Autodesk Inventor part; units mm, degrees
ref_plane "scharnier_XY" through (0, -8.75, 0) normal (0, 0, 1) x (1, 0, 0)
ref_plane "scharnier_YZ" through (0, -8.75, 0) normal (1, 0, 0) x (0, 1, 0)
ref_plane "scharnier_ZX" through (0, -8.75, 0) normal (0, 1, 0) x (0, 0, 1)
sketch "Skizze_1" plane through (0, 0, 0) normal (0, 1, 0) x (-1, 0, 0)
  arc A0 (9, 5.9981) -> (8.3959, 7.8036) centre (6, 5.9981) ccw
  line L0 (8.3959, 7.8036) -> (4.8967, 12.4471)
  arc A1 (4.8967, 12.4471) -> (3.9166, 13.2866) centre (2.5008, 10.6417) ccw
  line L1 (3.9166, 13.2866) -> (-0.1415, 15.4588)
  arc A2 (-0.1415, 15.4588) -> (2.0342, 12.1617) centre (-2.1, 11.8) ccw
  line L2 (2.0342, 12.1617) -> (0.5399, 12.031)
  arc A3 (-0.8494, 14.1363) -> (0.5399, 12.031) centre (-2.1, 11.8) ccw
  line L3 (-0.8494, 14.1363) -> (3.5, 11.8082)
  line L4 (3.5, 11.8082) -> (7.5, 6.5)
  line L5 (7.5, 6.5) -> (7.5, 3)
  arc A4 (6, 1.5) -> (7.5, 3) centre (6, 3) ccw
  line L6 (6, 1.5) -> (-5.3, 1.5)
  line L7 (-5.3, 1.5) -> (-6, 0.8)
  line L8 (-6, 0.8) -> (-6, 0)
  line L9 (-6, 0) -> (6, 0)
  arc A5 (6, 0) -> (9, 3) centre (6, 3) ccw
  line L10 (9, 3) -> (9, 5.9981)
extrude "Extrusion1" add sketch "Skizze_1" along normal mid plane 60
sketch "Skizze_2" plane through (0, 0, 0) normal (1, 0, 0) x (0, 1, 0)
  line L0 (8.75, 0) -> (8.75, 1.5)
  line L1 (8.75, 1.5) -> (12.35, 1.5)
  line L2 (12.35, 1.5) -> (10.85, 0)
  line L3 (10.85, 0) -> (8.75, 0)
  line L4 (8.75, 0) -> (8.75, 1.5)
revolve "Revolution1" cut sketch "Skizze_2" angle 360 about axis through (0, 8.75, 0) along (0, 0, -1)
sketch "Skizze_3" plane through (0, 0, 0) normal (1, 0, 0) x (0, 1, 0)
  line L0 (-8.75, 0) -> (-8.75, 1.5)
  line L1 (-8.75, 1.5) -> (-5.15, 1.5)
  line L2 (-5.15, 1.5) -> (-6.65, 0)
  line L3 (-6.65, 0) -> (-8.75, 0)
  line L4 (-8.75, 0) -> (-8.75, 1.5)
revolve "Revolution2" cut sketch "Skizze_3" angle 360 about axis through (0, -8.75, 0) along (0, 0, -1)
sketch "Skizze_5" plane through (0, 0, 0) normal (0, 1, 0) x (-1, 0, 0)
  line L0 (19.1684, 40) -> (-42.1, 40)
  line L1 (-42.1, 40) -> (-42.1, 3)
  line L2 (-42.1, 3) -> (-0.5049, 3)
  line L3 (-0.5049, 3) -> (19.1684, 40)
extrude "Extrusion2" cut sketch "Skizze_5" along normal mid plane 26
ref_plane "scharnier_XY" through (0, -8.75, 0) normal (0, 0, 1) x (1, 0, 0)
ref_plane "scharnier_YZ" through (0, -8.75, 0) normal (1, 0, 0) x (0, 1, 0)
ref_plane "scharnier_ZX" through (0, -8.75, 0) normal (0, 1, 0) x (0, 0, 1)
ref_plane "scharnier_2_XY" through (0, 8.75, 0) normal (0, 0, 1) x (1, 0, 0)
ref_plane "scharnier_2_YZ" through (0, 8.75, 0) normal (1, 0, 0) x (0, 1, 0)
ref_plane "scharnier_2_ZX" through (0, 8.75, 0) normal (0, 1, 0) x (0, 0, 1)
ref_plane "tuer_XY" through (2.1, 0, 11.8) normal (0, 1, 0) x (1, 0, 0)
ref_plane "tuer_YZ" through (2.1, 0, 11.8) normal (1, 0, 0) x (0, 0, -1)
ref_plane "tuer_ZX" through (2.1, 0, 11.8) normal (0, 0, -1) x (0, 1, 0)
properties part number "1XXX_01_04"
The model under review builds one solid part; all positions refer to its coordinate system, in mm. A direction names the side the tool comes from. Give positions to 0.01 mm unless a question says otherwise; leave off trailing zeros. Write each loop counter-clockwise with the first axis right and the second up, starting at its lowest first coordinate (ties: lowest second). Pieces come first, ordered by that corner, then holes.
1. Add section B-B, the plane z = 9.75. Write out the cut boundary in (x, y).
2. Add section A-A, the plane y = -8.75. Write out the cut boundary in (x, z).
3. Add section C-C, the plane y = 14. Write out the cut boundary in (x, z), plus the area to 3 significant figures.
4. Tool access review of faces 4 (the flat face through (-6.671, -0.42, 10.093)), 5 (the flat face through (-1.29, -21.62, 12.99)), 6 (the flat face through (0, 0, 0)), 7 (the flat face through (0, 0, 1.5)), 8 (the flat face through (-4.275, -0.182, 11.99)): name each direction out of +Z, -Z, +X, -X, +Y, -Y from which nothing blocks a thin tool from reaching the whole face with its end or side.
5. Wall thickness on L1, parallel to Y at x = 5.25, z = 9.75; L2, parallel to X at y = -18, z = 10.75; L3, parallel to Z at x = 4.5, y = -24.5: over which ranges is each line inside the solid? List them lowest first.
6. Draft analysis for pull direction Y (two halves, no side actions). For faces 1 (the flat face through (-0.8, -30, 9.2)), 2 (the flat face through (0, -13, 14)), 3 (the cylindrical face through (5.48, 21.38, 9.39)), state which applies: +Y half, -Y half, draft (parallel to the pull), parting line (faces both ways), or undercut.
7. For P1, Ø1, axis at y = 6.5, z = 5, coming from the +X side; P2, Ø0.6, axis at y = -3, z = 0.5, coming from the +X side; P3, Ø3.5, axis at x = -0.5, y = 3, coming from the +Z side, all flat-tipped, find the tip position at first contact; note any pin that passes through.
Worked answers:
1. outline: (-6.93, -30) - (-5.05, -30) - (-5.05, 30) - (-6.93, 30) - close; (-1.51, -30) - (0.42, -30) - (0.42, -13) - (-1.51, -13) - close; (-1.51, 13) - (0.42, 13) - (0.42, 30) - (-1.51, 30) - close; (3.78, -30) - (5.71, -30) - (5.71, -13) - (3.78, -13) - close; (3.78, 13) - (5.71, 13) - (5.71, 30) - (3.78, 30) - close
2. outline: (-9, 3) arc R3 ccw to (-6, 0) - (-2.1, 0) - (-3.6, 1.5) - (-6, 1.5) arc R1.5 cw to (-7.5, 3) - (-7.5, 6.5) - (-3.9, 11.28) - (-4.66, 12.72) arc R3 ccw to (-4.9, 12.45) - (-8.4, 7.8) arc R3 ccw to (-9, 6) - close; (2.1, 0) - (6, 0) - (6, 0.8) - (5.3, 1.5) - (3.6, 1.5) - close
3. outline: (-9, 3) arc R3 ccw to (-6, 0) - (6, 0) - (6, 0.8) - (5.3, 1.5) - (-6, 1.5) arc R1.5 cw to (-7.5, 3) - (-7.5, 6.5) - (-3.5, 11.81) - (0.85, 14.14) arc R2.65 cw (long way) to (-0.54, 12.03) - (-2.03, 12.16) arc R4.15 ccw (long way) to (0.14, 15.46) - (-3.92, 13.29) arc R3 ccw to (-4.9, 12.45) - (-8.4, 7.8) arc R3 ccw to (-9, 6) - close
3. area: 73.8 mm2
4. face 4: +Z, -X, +Y, -Y
4. face 5: +Y, -Y
4. face 6: -Z, +X, -X, +Y, -Y
4. face 7: +X, +Y, -Y
4. face 8: +Z, +X
5. L1: y = -30 to -13, 13 to 30
5. L2: x = -6.18 to -4.3, -1.91 to -0.33, 4.53 to 6.11
5. L3: z = 0 to 1.5, 8.41 to 10.68, 12.92 to 15.19
6. face 1: -Y half
6. face 2: undercut
6. face 3: draft
7. P1: stops at x = -7.5
7. P2: stops at x = 6
7. P3: stops at z = 1.5
